Input: part model. Units: mm. Frame: model coordinates. A direction names the side the tool comes from. Round coordinates to 2 decimals unless told otherwise and drop trailing zeros. Write each loop counter-clockwise with the first axis right and the second up, starting at its lowest first coordinate (ties: lowest second). Pieces come first, ordered by that corner, then holes. Notation, with made-up numbers: (8.25, -5.75) -> (41.25, -5.75) arc R11 ccw to (41.25, 2.25) -> close; hole circle Ø1 at (63, 31.5). An arc over 180 degrees is marked (long way). Write item = value, one per line.
```python
from build123d import *

# Parameters (mm, degrees)
BOSS_EXTRUDE1_DEPTH = 22.86
SKETCH2_R           = 2.413
CUT_EXTRUDE1_DEPTH  = 54.73826082
SKETCH3_R           = 2.413
CUT_EXTRUDE2_DEPTH  = 54.55787408
CHAMFER1_SIZE       = 6.35


with BuildPart() as part:
    # Sketch1 → Boss-Extrude1 (new body)
    with BuildSketch(Plane(origin=(0, 0, 0), x_dir=(1, 0, 0), z_dir=(0, 1, 0))):
        Polygon((0, 0), (0, 38.1), (31.75, 38.1), (31.75, 36.576), (1.524, 36.576), (1.524, 0), align=None)
    extrude(amount=BOSS_EXTRUDE1_DEPTH)

    # Sketch2 → Cut-Extrude1 (cut, through all)
    with BuildSketch(Plane(origin=(1.524, 0, 0), x_dir=(0, 0, -1), z_dir=(1, 0, 0))):
        with Locations((6.35, 12.7)):
            Circle(SKETCH2_R)
        with Locations((19.05, 12.7)):
            Circle(SKETCH2_R)
    extrude(amount=-CUT_EXTRUDE1_DEPTH, mode=Mode.SUBTRACT)

    # Sketch3 → Cut-Extrude2 (cut, through all)
    with BuildSketch(Plane.XY.offset(-36.576)):
        with Locations((25.4, 12.7)):
            Circle(SKETCH3_R)
        with Locations((12.7, 12.7)):
            Circle(SKETCH3_R)
    extrude(amount=-CUT_EXTRUDE2_DEPTH, mode=Mode.SUBTRACT)

    # Chamfer1
    chamfer1_edges = [part.edges().sort_by_distance(p)[0] for p in [
        (31.75, 22.86, -37.338),
        (0.762, 22.86, 0),
        (31.75, 0, -37.338),
        (0.762, 0, 0),
    ]]
    chamfer(chamfer1_edges, length=CHAMFER1_SIZE)


solid = part.part
```
1) Access query for faces 1 (the face through (16, 11, -38.1)), 2 (the face through (17, 11, -36.576)). Directions: +Z, -Z, +X, -X, +Y, -Y. A direction counts if a zero-diameter tool reaches every point of the face in a straight line with its end or side. Return the directions, or none.
Solutions:
face_1 = -Z, +X, -X, +Y, -Y
face_2 = +Z, +X, +Y, -Y
2) Cut plane B-B (x = 12.7). Return the cut outline in (y, z), and give its area (3 significant figures).
Solutions:
outline = (0, -38.1) -> (10.29, -38.1) -> (10.29, -36.58) -> (0, -36.58) -> close; (15.11, -38.1) -> (22.86, -38.1) -> (22.86, -36.58) -> (15.11, -36.58) -> close
area = 27.5 mm^2
3) Cut plane D-D (y = 5.5). Return the cut outline in (x, z), and give its area (3 significant figures).
Solutions:
outline = (0, -38.1) -> (30.9, -38.1) -> (30.9, -36.58) -> (1.52, -36.58) -> (1.52, -0.85) -> (0, -0.85) -> close
area = 102 mm^2
4) Cut plane C-C (y = 12.7). Return the cut outline in (x, z), and give its area (3 significant figures).
Solutions:
outline = (0, -38.1) -> (10.29, -38.1) -> (10.29, -36.58) -> (1.52, -36.58) -> (1.52, -21.46) -> (0, -21.46) -> close; (0, -16.64) -> (1.52, -16.64) -> (1.52, -8.76) -> (0, -8.76) -> close; (0, -3.94) -> (1.52, -3.94) -> (1.52, 0) -> (0, 0) -> close; (15.11, -38.1) -> (22.99, -38.1) -> (22.99, -36.58) -> (15.11, -36.58) -> close; (27.81, -38.1) -> (31.75, -38.1) -> (31.75, -36.58) -> (27.81, -36.58) -> close
area = 74.7 mm^2
5) First-contact query: P1, Ø6.5, axis at y = 12.7, z = -6.35, coming from the -X side; P2, Ø3, axis at x = 12.7, y = 12.7, coming from the +Z side; P3, Ø6.5, axis at y = 12.7, z = -19.05, coming from the +X side; P4, Ø11.5, axis at x = 20.5, y = 11.5, coming from the +Z side. Flat tips, straight axial feed; report the tip coordinate or a pass-through.
Solutions:
P1 = 0
P2 = through
P3 = 1.52
P4 = -36.58
6) Line query: L1, parallel to Y at x = 0.7, z = -6.35; L2, parallel to Z at x = 5, y = 7.5; L3, parallel to X at y = 9.25, z = -10.5. Output: solid intervals per line, ascending. Write a range as from..to.
Solutions:
L1 = 0..10.29, 15.11..22.86
L2 = -38.1..-36.58
L3 = 0..1.52
7) Draft query along Y for faces 3 (the face through (0, 9, -19)), 4 (the face through (0.773, 10.559, -7.463)), 5 (the face through (0.77, 19.73, -3.22)). Return one class per face: +Y half, -Y half, draft (parallel to the pull), parting line (faces both ways), or undercut.
Solutions:
face_3 = draft
face_4 = undercut
face_5 = +Y half
8) Cut plane A-A (z = -19.05). Return the cut outline in (x, y).
Solutions:
outline = (0, 0) -> (1.52, 0) -> (1.52, 10.29) -> (0, 10.29) -> close; (0, 15.11) -> (1.52, 15.11) -> (1.52, 22.86) -> (0, 22.86) -> close
